Build history of the part. All positions in model axes, mm. A direction names the side the tool comes from. Round coordinates to 2 decimals unless told otherwise and drop trailing zeros. Write each loop counter-clockwise with the first axis right and the second up, starting at its lowest first coordinate (ties: lowest second). Pieces come first, ordered by that corner, then holes.
1) Wall check: probe 1 along X at (y, z) = (86.5, 6.25); probe 2 along Y at (x, z) = (7, 2.75); probe 3 along Y at (x, z) = (-2.5, 0.5). Give the ranges that are in metal, low to high.
2) Saw through at A-A (y = 64). Write the cut outline in (x, z), plus the area to 3 significant figures.
3) Saw through at C-C (z = 5). Write the cut outline in (x, y).
4) Flat gauge pins, fed straight in: pin 1 (4 mm diameter, centred on x = 33.5, z = 1.5, fed in from -Y); pin 2 (5 mm diameter, centred on x = -10.5, z = 6.5, fed in from +Y); pin 3 (3 mm diameter, centred on y = 81, z = 4, fed in from +X). Where does each tip first touch, or does it go through?
5) Which spindle directions (+Z, -Z, +X, -X, +Y, -Y) get a long thin tool onto all of the face, cutting with end or side? Do faces 1 (the flat face through (0, 82, 5)), 2 (the flat face through (23, 82, 5)), 3 (the flat face through (-12, 57, 5)), 4 (the cylindrical face through (9, -5, 5)), 5 (the flat face through (34, 57, 5)). Say none if no direction does.
6) Saw through at D-D (x = 11.5). Write the cut outline in (y, z).
7) Pull direction X, two halves, no side cores. Call faces 6 (the cylindrical face through (-1.33, 66.48, 5.07)), 7 (the flat face through (23, 28, 5)), 8 (the flat face through (-11, 72, 5)): +X half, -X half, draft (parallel to the pull), parting line (faces both ways), or undercut.
8) Saw through at B-B (x = 24). Write the cut outline in (y, z), plus the area to 3 significant figures.
from build123d import *

# Parameters (mm, degrees)
PAD_DEPTH    = 10
SKETCH001_R  = 2.5
PAD001_DEPTH = 10
SKETCH002_R  = 2.5
POCKET_DEPTH = 10


with BuildPart() as part:
    # Sketch → Pad (new body)
    with BuildSketch(Plane.XY):
        Polygon((0, 0), (23, 0), (23, 57), (46, 57), (46, 72), (23, 72), (23, 92), (0, 92), (0, 72), (-23, 72), (-23, 57), (0, 57), align=None)
    extrude(amount=PAD_DEPTH)

    # Sketch001 → Pad001 (new body)
    with BuildSketch(Plane.XZ):
        with Locations((11.5, 5)):
            Circle(SKETCH001_R)
    extrude(amount=PAD001_DEPTH)

    # Sketch002 → Pocket (cut)
    with BuildSketch(Plane.XY.offset(10)):
        with Locations((24, 64)):
            Circle(SKETCH002_R)
        with Locations((-1, 64)):
            Circle(SKETCH002_R)
    extrude(amount=-POCKET_DEPTH, mode=Mode.SUBTRACT)


solid = part.part
Evaluation:
1. probe 1: x = 0 to 23
1. probe 2: y = 0 to 92
1. probe 3: y = 57 to 62, 66 to 72
2. outline: (-23, 0) - (-3.5, 0) - (-3.5, 10) - (-23, 10) - close; (1.5, 0) - (21.5, 0) - (21.5, 10) - (1.5, 10) - close; (26.5, 0) - (46, 0) - (46, 10) - (26.5, 10) - close
2. area: 590 mm2
3. outline: (-23, 57) - (0, 57) - (0, 0) - (9, 0) - (9, -10) - (14, -10) - (14, 0) - (23, 0) - (23, 57) - (46, 57) - (46, 72) - (23, 72) - (23, 92) - (0, 92) - (0, 72) - (-23, 72) - close; hole circle Ø5 at (-1, 64); hole circle Ø5 at (24, 64)
4. pin 1: stops at y = 57
4. pin 2: stops at y = 72
4. pin 3: stops at x = 23
5. face 1: +Z, -Z, -X, +Y
5. face 2: +Z, -Z, +X, +Y
5. face 3: +Z, -Z, -X, -Y
5. face 4: -Y
5. face 5: +Z, -Z, +X, -Y
6. outline: (-10, 2.5) - (0, 2.5) - (0, 0) - (92, 0) - (92, 10) - (0, 10) - (0, 7.5) - (-10, 7.5) - close
7. face 6: undercut
7. face 7: +X half
7. face 8: draft
8. outline: (57, 0) - (61.5, 0) - (61.5, 10) - (57, 10) - close; (66.5, 0) - (72, 0) - (72, 10) - (66.5, 10) - close
8. area: 100 mm2
